The figure shows three views and two pictorial views of one solid part (mm, origin at its lowest corner). Answer the questions. Coordinates: 2 decimals unless noted, no trailing zeros. Order: outer loops, then holes, each group sorted by start corner. A loop starts at its lowest first (then second) coordinate and runs counter-clockwise, first axis right, second up. Notation, with made-up numbers: (-26.75, 68.5) -> (22.25, 68.5) arc R9 ccw to (22.25, 85.5) -> close; hole circle Ø10 at (12, 61). An arc over 180 degrees is marked (long way). Return JSON: item names as keys, results as strings. Group by question number.
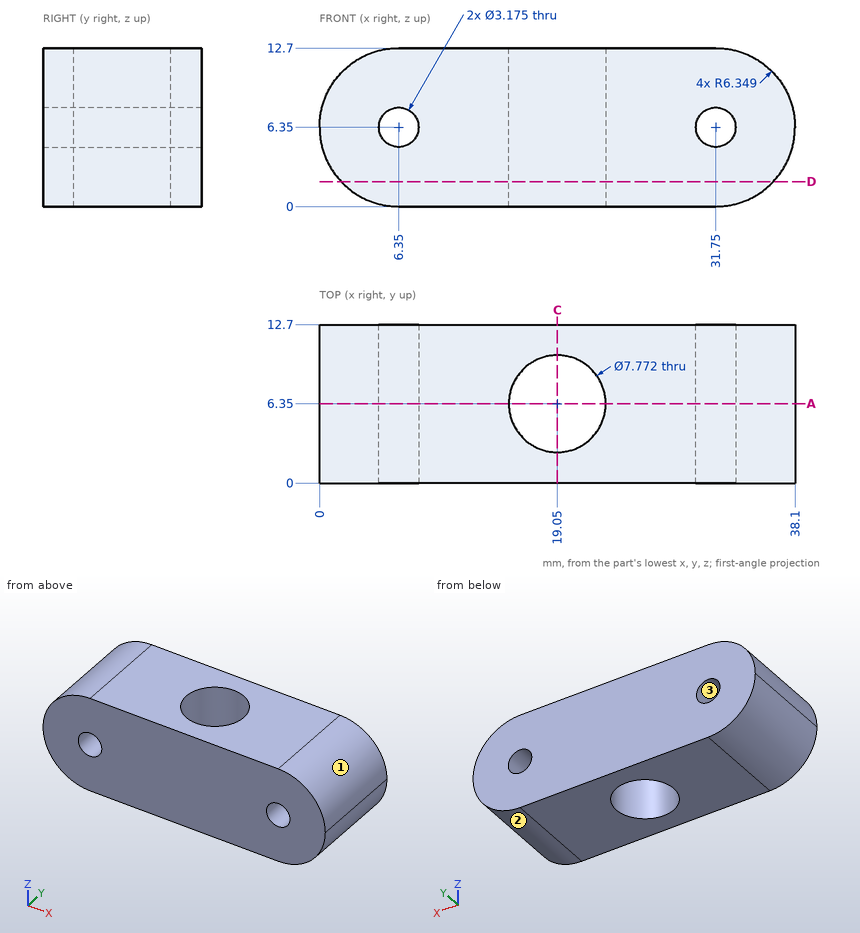
1. Find section C-C on x = 19.05. Determine the outline of the cut face in (y, z).
2. Straight lines are drawn through the part: L1, parallel to Z at x = 31.75, y = 6.75; L2, parallel to Y at x = 19.05, z = 10; L3, parallel to X at y = 11.75, z = 5 (1 decimal). For each, find the intervals that lie inside material, in ascending order.
3. Find section D-D on z = 2. Determine the outline of the cut face in (x, y).
4. Given pin 1 (7 mm diameter, centred on x = 19.05, y = 6.35, fed in from +Z); pin 2 (1 mm diameter, centred on y = 7.5, z = 4, fed in from -X) (1 decimal), each flat-ended and moving along its own axis, determine where each tip first touches the part or whether it passes through.
5. For a pull along Z with two mould halves and no side action, classify the marked faces 1, 2 and 3 as released by +Z, released by -Z, zero draft, split by the parting line, or undercut.
6. Find section A-A on y = 6.35. Give the number of separate pieces and of enclosed holes in the cut face, and give its area (3 significant figures).
Result:
{
 "1": {"outline": "(0, 0) -> (2.46, 0) -> (2.46, 12.7) -> (0, 12.7) -> close; (10.24, 0) -> (12.7, 0) -> (12.7, 12.7) -> (10.24, 12.7) -> close"},
 "2": {"L1": "0 to 4.76, 7.94 to 12.7", "L2": "0 to 2.46, 10.24 to 12.7", "L3": "0.1 to 5.5, 7.2 to 30.9, 32.6 to 38"},
 "3": {"outline": "(1.72, 0) -> (36.38, 0) -> (36.38, 12.7) -> (1.72, 12.7) -> close; hole circle Ø7.77 at (19.05, 6.35)"},
 "4": {"pin 1": "through", "pin 2": "x = 0.3"},
 "5": {"face 1": "released by +Z", "face 2": "released by -Z", "face 3": "undercut"},
 "6": {"separate pieces": "2", "enclosed holes": "2", "area": "335 mm^2"}
}
